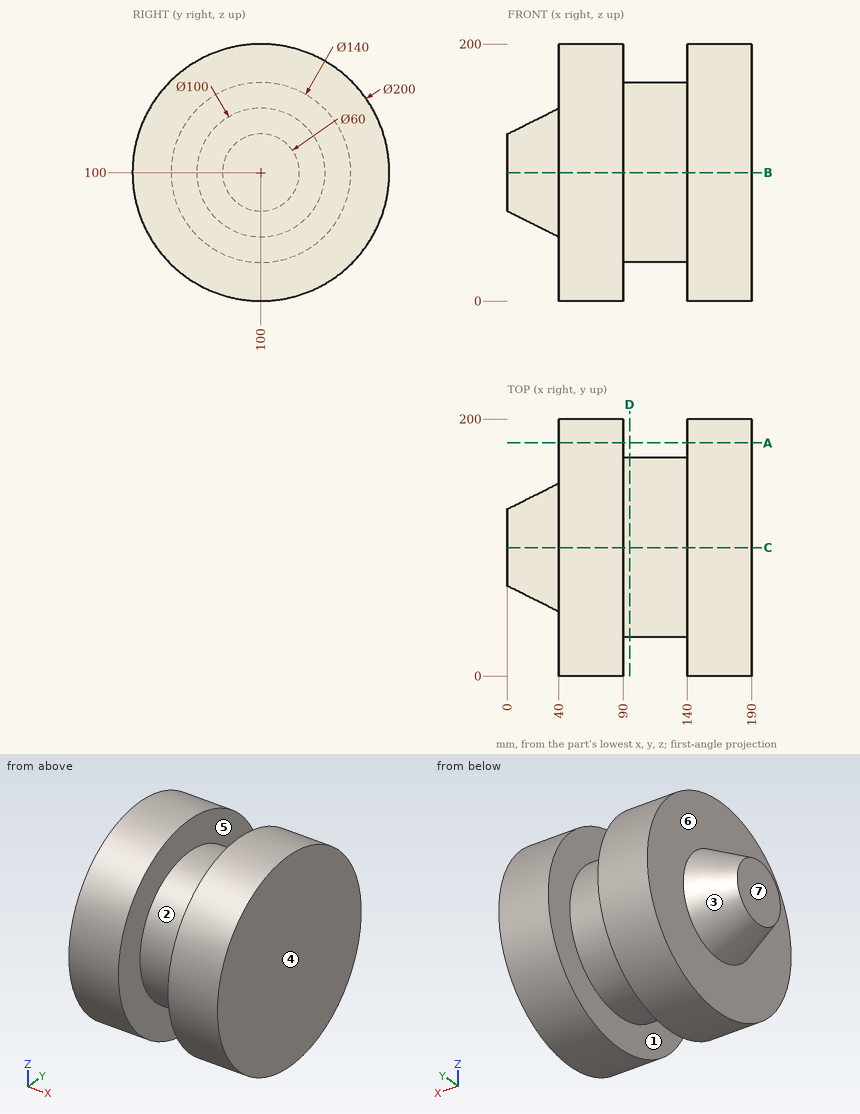
The drawing under review shows one solid part. Ordinate dimensions are in mm from its lowest x, y, z. A direction names the side the tool comes from. Round coordinates to 2 decimals unless told otherwise and drop trailing zeros. Write each loop counter-clockwise with the first axis right and the second up, starting at its lowest first coordinate (ties: lowest second). Pieces come first, ordered by that corner, then holes. Notation, with made-up numbers: (81.25, 41.25) - (130.25, 41.25) arc R20 cw to (130.25, 64.25) - close; hole circle Ø5 at (9, 39). An arc over 180 degrees is marked (long way). Write each question's results on one line, items separated by ' | '.
Item 1: Take a section at A-A on y = 181.5. State the section outline as (x, z) points.
Calculated:
outline: (40, 42.05) - (90, 42.05) - (90, 157.95) - (40, 157.95) - close; (140, 42.05) - (190, 42.05) - (190, 157.95) - (140, 157.95) - close
Item 2: Take a section at D-D on x = 95. State the section outline as (y, z) points, then the cut area to 3 significant figures.
Calculated:
outline: circle Ø140 at (100, 100) | area: 15,400 mm^2
Item 3: To check wall thickness, follow line 1 along X through (y, z) = (98.5, 184); line 2 along Y through (x, z) = (71, 103.5); line 3 along X through (y, z) = (139, 66). State the ranges of each line that lie inside material, in increasing order. Write a range as from..to.
Calculated:
line 1: x = 40..90, 140..190 | line 2: y = 0.06..199.94 | line 3: x = 40..190
Item 4: For the marked faces 5, 6 and 7, list the 3-axis set-ups (+Z, -Z, +X, -X, +Y, -Y) from which the entire face can be reached by the end or side of a thin tool; tool diameter is ignored.
Calculated:
face 5: none | face 6: -X | face 7: +Z, -Z, -X, +Y, -Y
Item 5: Draft analysis for pull direction X (two halves, no side actions). For the marked faces 1, 2, 3 and 4, state which applies: pulls with the +X half, pulls with the -X half, needs draft (parallel to the pull), parting line crosses it, or undercut.
Calculated:
face 1: undercut | face 2: undercut | face 3: pulls with the -X half | face 4: pulls with the +X half
Item 6: Take a section at B-B on z = 100. State the section outline as (x, y) points.
Calculated:
outline: (0, 70) - (40, 50) - (40, 0) - (90, 0) - (90, 30) - (140, 30) - (140, 0) - (190, 0) - (190, 200) - (140, 200) - (140, 170) - (90, 170) - (90, 200) - (40, 200) - (40, 150) - (0, 130) - close
Item 7: For pin 1 (1 mm diameter, centred on y = 97, z = 66.5, fed in from -X); pin 2 (2 mm diameter, centred on x = 152, z = 68, fed in from -Y); pin 3 (6 mm diameter, centred on x = 170.5, z = 148, fed in from +Y), all flat-tipped, find the tip position at first contact; note any pin that passes through.
Calculated:
pin 1: stops at x = 6.27 | pin 2: stops at y = 4.93 | pin 3: stops at y = 189.3
